Can you work these out from the model? Positions are in its coordinate system, mm. A direction names the side the tool comes from. Give positions to 0.01 mm unless a question says otherwise; leave off trailing zeros. Loops run counter-clockwise (first coordinate to the right, second up) from the corner with the lowest first, then second, coordinate; pieces in that order, holes last. Notation, with made-up numbers: (70, -32.75) -> (87, -32.75) arc R8 cw to (87, -22.75) -> close; hole circle Ø2 at (46.5, 67). An arc over 180 degrees is marked (long way). Return JSON: item names as keys, results as strings. Group by question number.
Q1. Will these pins go through, and if not, where does the flat tip stop? pin 1 (2 mm diameter, centred on y = 15.5, z = 18.5, fed in from -X); pin 2 (11 mm diameter, centred on y = 21, z = 18, fed in from -X); pin 3 (11 mm diameter, centred on x = -17, z = 12, fed in from +Y).
Q2. Suppose I cut it at C-C, the plane y = 11.5. Please give me the cut outline in (x, z), and give its area (4 significant figures).
Q3. Suppose I cut it at D-D, the plane x = -17. Please give me the cut outline in (y, z).
Q4. Which directions (+Z, -Z, +X, -X, +Y, -Y) give clear straight access to the entire face, cutting with the end or side of a thin tool? Please do faces 1 (the flat face through (-20, 3, 12)), 2 (the flat face through (-20, 14, 21)), 3 (the flat face through (-20, 16, 4)), 4 (the flat face through (-15, 10, 0)).
Q5. Suppose I cut it at B-B, the plane z = 17.75. Please give me the cut outline in (x, y).
Q6. Suppose I cut it at A-A, the plane y = 2. Please give me the cut outline in (x, z).
Q7. I need wall thicknesses on line 1 along X through (y, z) = (3.25, 23.25); line 2 along X through (y, z) = (22.5, 14.75); line 3 along Y through (x, z) = (-13.75, 8.75). Which ranges of each line are inside material? Lowest first, please. Write a range as [from, to].
```python
from build123d import *

# Parameters (mm, degrees)
BOSS_EXTRUDE1_DEPTH = 25
BOSS_EXTRUDE2_DEPTH = 10


with BuildPart() as part:
    # Sketch1 → Boss-Extrude1 (new body)
    with BuildSketch(Plane.XY):
        Polygon((-30, 10), (-20, 10), (-20, 15), (-10, 15), (-10, 25), (0, 25), (0, 0), (-10, 0), (-10, 5), (-20, 5), (-20, 0), (-30, 0), align=None)
    extrude(amount=BOSS_EXTRUDE1_DEPTH)

    # Sketch2 → Boss-Extrude2 (add)
    with BuildSketch(Plane.ZY.offset(20)):
        Polygon((0, 10), (0, 20), (25, 10), align=None)
    extrude(amount=BOSS_EXTRUDE2_DEPTH)


solid = part.part
```
Ans:
{
 "1": {"pin 1": "stops at x = -20", "pin 2": "stops at x = -10", "pin 3": "stops at y = 17.04"},
 "2": {"outline": "(-30, 0) -> (0, 0) -> (0, 25) -> (-20, 25) -> (-20, 21.25) -> (-30, 21.25) -> close", "area": "712.5 mm^2"},
 "3": {"outline": "(5, 0) -> (15, 0) -> (15, 25) -> (5, 25) -> close"},
 "4": {"face 1": "+Z, -Z, -Y", "face 2": "+Z, -X, +Y", "face 3": "+Z, -Z, +Y", "face 4": "-Z, +X, -X, +Y, -Y"},
 "5": {"outline": "(-30, 0) -> (-20, 0) -> (-20, 5) -> (-10, 5) -> (-10, 0) -> (0, 0) -> (0, 25) -> (-10, 25) -> (-10, 15) -> (-20, 15) -> (-20, 12.9) -> (-30, 12.9) -> close"},
 "6": {"outline": "(-30, 0) -> (-20, 0) -> (-20, 25) -> (-30, 25) -> close; (-10, 0) -> (0, 0) -> (0, 25) -> (-10, 25) -> close"},
 "7": {"line 1": "x = [-30, -20], [-10, 0]", "line 2": "x = [-10, 0]", "line 3": "y = [5, 15]"}
}
